from build123d import *

# Parameters (mm, degrees)
F0_W     = 242.7079752088
F0_H     = 38.4193509817
F1_DEPTH = 185.928
F2_R     = 28.5688993419
F3_DEPTH = 122.174
F4_R     = 8.5256392181
F4_R_2   = 7.1835260989
F4_R_3   = 5.0238918194
F5_DEPTH = 110.744


with BuildPart() as f1:
    # F0 (on Front) → F1 (new body)
    with BuildSketch(Plane.XZ):
        with Locations((-4.9031935632, -51.0637238622)):
            Rectangle(F0_W, F0_H)
    extrude(amount=F1_DEPTH)

    # F2 (on face) → F3 (join)
    with BuildSketch(Plane.XY.offset(-31.8540483713)):
        with Locations((-12.5624807552, -87.5830799341)):
            Circle(F2_R)
    extrude(amount=F3_DEPTH)

    # F4 (on Front) → F5 (join)
    with BuildSketch(Plane.XZ):
        with BuildLine():
            Line((-31.2578417361, 0), (-81.515558064, 0))
            Line((-81.515558064, 0), (-81.515558064, -78.5908699036))
            Line((-81.515558064, -78.5908699036), (-31.2578417361, -78.5908699036))
            Line((-31.2578417361, -78.5908699036), (-31.2578417361, -68.2470542583))
            ThreePointArc((-31.2578417361, -68.2470542583), (-54.1109280597, -64.0015229583), (-31.2578417361, -59.7559916582))
            Line((-31.2578417361, -59.7559916582), (-31.2578417361, 0))
        make_face()
        with Locations((-68.0317804217, -68.9809322357)):
            Circle(F4_R, mode=Mode.SUBTRACT)
        with Locations((-72.3220780492, -30.3810052574)):
            Circle(F4_R_2, mode=Mode.SUBTRACT)
        with Locations((-47.1932142973, -37.2236035764)):
            Circle(F4_R_3, mode=Mode.SUBTRACT)
        with BuildLine():
            ThreePointArc((-30.4691283096, -64.0015229583), (-30.6679791986, -61.8424372207), (-31.2578417361, -59.7559916582))
            Line((-31.2578417361, -59.7559916582), (-31.2578417361, -68.2470542583))
            ThreePointArc((-31.2578417361, -68.2470542583), (-30.6679791986, -66.1606086959), (-30.4691283096, -64.0015229583))
        make_face()
        with BuildLine():
            Line((-31.2578417361, -68.2470542583), (-31.2578417361, -59.7559916582))
            ThreePointArc((-31.2578417361, -59.7559916582), (-54.1109280597, -64.0015229583), (-31.2578417361, -68.2470542583))
        make_face()
    extrude(amount=F5_DEPTH)


solid = f1.part
CAD build for the part. Positions are in the model's coordinates, mm. A direction names the side the tool comes from. Coordinates: 2 decimals unless noted, no trailing zeros. Order: outer loops, then holes, each group sorted by start corner. A loop starts at its lowest first (then second) coordinate and runs counter-clockwise, first axis right, second up.
Item 1: Two-plate mould, pull along X, no slides. Class faces 4 (the face through (-81.516, -55, -16)), 5 (the face through (-68.201, -54.597, -77.505)), 6 (the face through (116.451, -92, -51)): +X half, -X half, draft (parallel to the pull), parting line (faces both ways), or undercut.
Check sheet entries:
face 4: -X half
face 5: undercut
face 6: +X half
Item 2: Band-saw the part on C-C on x = -14. List the corners of the cut face in (y, z).
Check sheet entries:
outline: (-185.93, -70.27) - (0, -70.27) - (0, -31.85) - (-59.05, -31.85) - (-59.05, 90.32) - (-116.12, 90.32) - (-116.12, -31.85) - (-185.93, -31.85) - close
Item 3: Pin check, flat tips, straight feed: pin 1 Ø4 at (y, z) = (-97.5, 40.5) entering from +X; pin 2 Ø4 at (x, y) = (-58.5, -137) entering from -Z; pin 3 Ø10 at (x, y) = (18, -26.5) entering from +Z. Stop position of each tip, or through.
Check sheet entries:
pin 1: stops at x = 14.89
pin 2: stops at z = -70.27
pin 3: stops at z = -31.85
Item 4: Band-saw the part on D-D on y = -147.5. List the corners of the cut face in (x, z), plus the area to 3 significant figures.
Check sheet entries:
outline: (-126.26, -70.27) - (116.45, -70.27) - (116.45, -31.85) - (-126.26, -31.85) - close
area: 9,320 mm2
Item 5: Drill centre lines: L1, parallel to Z at x = -19, y = -17.5; L2, parallel to X at y = -29.5, z = -19; L3, parallel to X at y = -98, z = -29. Where is each one in solid material? Low to high.
Check sheet entries:
L1: z = -70.27 to -31.85
L2: x = -81.52 to -31.26
L3: x = -81.52 to -79.37, -65.27 to 14.04
Item 6: Band-saw the part on A-A on z = -28. List the corners of the cut face in (x, y), plus the area to 3 significant figures.
Check sheet entries:
outline: (-81.52, -110.74) - (-79.1, -110.74) - (-79.1, 0) - (-81.52, 0) - close; (-65.54, -110.74) - (-31.26, -110.74) - (-31.26, -109.19) arc R28.57 ccw (long way) to (-31.26, -65.98) - (-31.26, 0) - (-65.54, 0) - close
area: 6,330 mm2
Item 7: 3-axis set-ups, long thin cutter, end or side, ignore diameter. For faces 1 (the face through (-57, -110.744, -16)), 2 (the face through (-31.258, -55, -74)), 3 (the face through (-51, -110.744, -74)): which of +Z, -Z, +X, -X, +Y, -Y reach the whole face in a straight line?
Check sheet entries:
face 1: +Z, -X, -Y
face 2: -Z, +X, +Y, -Y
face 3: -Z, +X, -X, -Y
Item 8: Band-saw the part on B-B on y = -78.5. List the corners of the cut face in (x, z), plus the area to 3 significant figures.
Check sheet entries:
outline: (-126.26, -70.27) - (-81.52, -70.27) - (-81.52, -78.59) - (-31.26, -78.59) - (-31.26, -70.27) - (116.45, -70.27) - (116.45, -31.85) - (14.52, -31.85) - (14.52, 90.32) - (-39.65, 90.32) - (-39.65, 0) - (-81.52, 0) - (-81.52, -31.85) - (-126.26, -31.85) - close; hole (-79.35, -31.85) - (-65.29, -31.85) arc R7.18 ccw (long way) to start; hole (-76.46, -70.27) arc R8.53 ccw to (-59.6, -70.27) - close
area: 17,500 mm2
